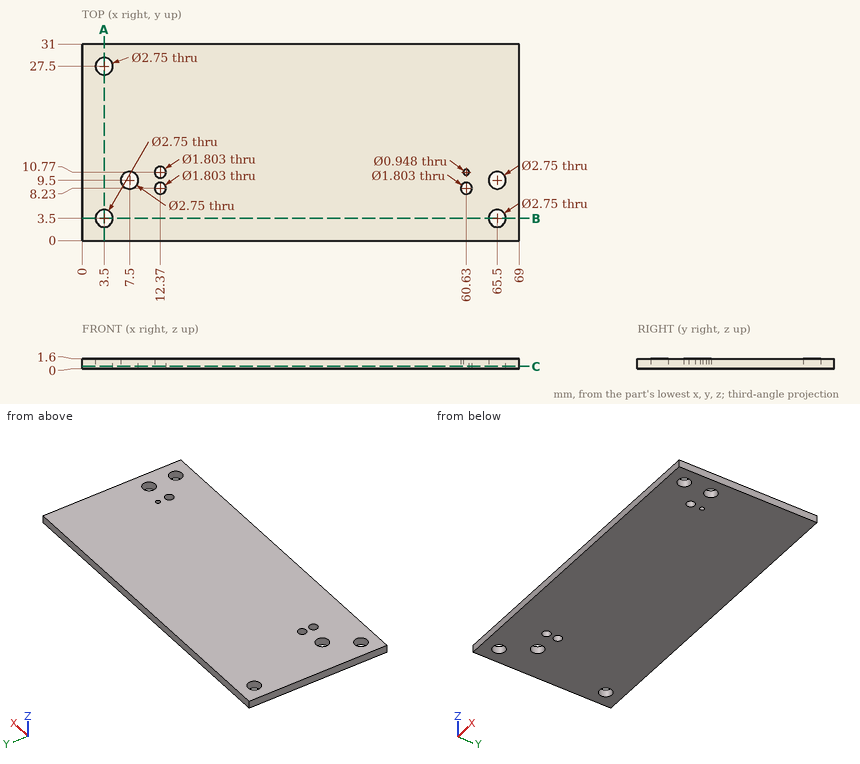
Design review of the part shown in the three views and the two pictorial views. Dimensions are in mm from the part's minimum x, y and z. Give positions to 0.01 mm unless a question says otherwise; leave off trailing zeros. Loops run counter-clockwise (first coordinate to the right, second up) from the corner with the lowest first, then second, coordinate; pieces in that order, holes last. Notation, with made-up numbers: (6.5, 31.25) -> (24.5, 31.25) arc R16 cw to (24.5, 50.25) -> close; hole circle Ø8 at (69.5, -28). An arc over 180 degrees is marked (long way). Put each result on its own line as item: value. Start each with the question number.
1. We need section A-A on x = 3.5. State the section outline as (y, z) points (3 decimals), then the cut area to 3 significant figures.
2. We need section B-B on y = 3.5. State the section outline as (x, z) points (3 decimals), then the cut area to 3 significant figures.
3. We need section C-C on z = 0.35. State how many separate pieces and enclosed holes the cut face has, then the cut area to 3 significant figures.
4. Wall thickness on probe 1 along Y at (x, z) = (60.63, 0.9); probe 2 along Y at (x, z) = (3.5, 0.45) (3 decimals); probe 3 along X at (y, z) = (10, 1.45): over which ranges is each line inside the solid? List them lowest first.
5. Clearance check with a flat-ended pin moving along its axis: P1, Ø2, axis at x = 7, y = 4.5, coming from the -Z side. State where the tip first meets the part, or that it passes through.
Determined:
1. outline: (0, 0) -> (2.125, 0) -> (2.125, 1.6) -> (0, 1.6) -> close; (4.875, 0) -> (26.125, 0) -> (26.125, 1.6) -> (4.875, 1.6) -> close; (28.875, 0) -> (31, 0) -> (31, 1.6) -> (28.875, 1.6) -> close
1. area: 40.8 mm^2
2. outline: (0, 0) -> (2.125, 0) -> (2.125, 1.6) -> (0, 1.6) -> close; (4.875, 0) -> (64.125, 0) -> (64.125, 1.6) -> (4.875, 1.6) -> close; (66.875, 0) -> (69, 0) -> (69, 1.6) -> (66.875, 1.6) -> close
2. area: 102 mm^2
3. separate pieces: 1
3. enclosed holes: 9
3. area: 2,100 mm^2
4. probe 1: 0 to 7.33, 9.13 to 10.3, 11.24 to 31
4. probe 2: 0 to 2.125, 4.875 to 26.125, 28.875 to 31
4. probe 3: 0 to 6.22, 8.78 to 11.9, 12.84 to 64.22, 66.78 to 69
5. P1: z = 0
